from build123d import *

# Parameters (mm, degrees)
EXTRUDE_1_DEPTH     = 191
SKETCH_2_R          = 4.25
CUT_EXTRUDE_1_DEPTH = 21
SKETCH_3_R          = 2.25
CUT_EXTRUDE_2_DEPTH = 41


with BuildPart() as part:
    # Эскиз1 → Бобышка-Вытянуть1 (new body)
    with BuildSketch(Plane(origin=(0, 0, 0), x_dir=(1, 0, 0), z_dir=(0, 1, 0))):
        Polygon((0, 0), (0, 20), (2, 20), (2, 2), (40, 2), (40, 0), align=None)
    extrude(amount=EXTRUDE_1_DEPTH)

    # Эскиз2 → Вырез-Вытянуть1 (cut, through all)
    with BuildSketch(Plane.XY):
        with Locations((20, 165.5)):
            Circle(SKETCH_2_R)
        with Locations((20, 95.5)):
            Circle(SKETCH_2_R)
        with Locations((20, 25.5)):
            Circle(SKETCH_2_R)
    extrude(amount=-CUT_EXTRUDE_1_DEPTH, mode=Mode.SUBTRACT)

    # Эскиз3 → Вырез-Вытянуть2 (cut, through all)
    with BuildSketch(Plane.ZY):
        with Locations((-10, 12)):
            Circle(SKETCH_3_R)
        with Locations((-10, 179)):
            Circle(SKETCH_3_R)
    extrude(amount=-CUT_EXTRUDE_2_DEPTH, mode=Mode.SUBTRACT)


solid = part.part
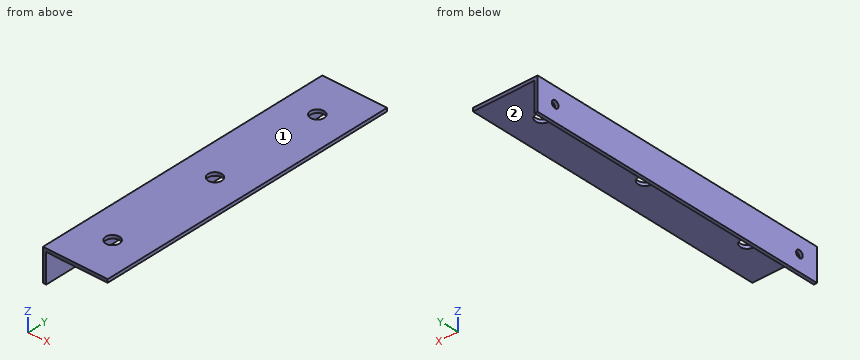
Geometry: final body of the model. Coordinates: model frame, mm. Face numbers are marked on the shaded views. A direction names the side the tool comes from. Coordinates: 2 decimals unless noted, no trailing zeros. Loops run counter-clockwise (first coordinate to the right, second up) from the corner with the lowest first, then second, coordinate; pieces in that order, holes last. Notation, with made-up numbers: M 2.25,-35.75 L 51.25,-35.75 A20 cw 51.25,-31.75 Z; hole C 60,0 d7. An arc over 180 degrees is marked long. One line per item, written item: value. Start each with the question number.
1) Pin query (flat end, axial travel): P1, Ø11, axis at x = 20, y = 25.5, coming from the -Z side; P2, Ø9, axis at y = 119.5, z = -12, coming from the +X side. Return the tip coordinate at first contact, or that it passes through.
2) Cut plane D-D (y = 88). Return loops of the section in (x, z), then the cut area to 3 significant figures.
3) Cut plane A-A (x = 20). Return loops of the section in (y, z).
4) Cut plane B-B (y = 179). Return loops of the section in (x, z), then the cut area to 3 significant figures.
5) Reachability of the marked faces 1 and 2 from +Z, -Z, +X, -X, +Y, -Y: full face, straight path, thin tool, end or side. Return the list, or none.
6) Material intervals for L1, parallel to Y at x = 1.35, z = -10; L2, parallel to Y at x = 20, z = -0.7; L3, parallel to X at y = 121, z = -17.25, sorted ascending. Write a range as from..to.
7) Cut plane C-C (z = -10). Return loops of the section in (x, y).
Evaluation:
1. P1: z = -2
1. P2: x = 2
2. outline: M 0,-20 L 2,-20 L 2,-2 L 40,-2 L 40,0 L 0,0 Z
2. area: 116 mm^2
3. outline: M 0,-2 L 21.25,-2 L 21.25,0 L 0,0 Z; M 29.75,-2 L 91.25,-2 L 91.25,0 L 29.75,0 Z; M 99.75,-2 L 161.25,-2 L 161.25,0 L 99.75,0 Z; M 169.75,-2 L 191,-2 L 191,0 L 169.75,0 Z
4. outline: M 0,-20 L 2,-20 L 2,-12.25 L 0,-12.25 Z; M 0,-7.75 L 2,-7.75 L 2,-2 L 40,-2 L 40,0 L 0,0 Z
4. area: 107 mm^2
5. face 1: +Z, +X, -X, +Y, -Y
5. face 2: -Z, +X, +Y, -Y
6. L1: 0..9.75, 14.25..176.75, 181.25..191
6. L2: 0..21.25, 29.75..91.25, 99.75..161.25, 169.75..191
6. L3: 0..2
7. outline: M 0,0 L 2,0 L 2,9.75 L 0,9.75 Z; M 0,14.25 L 2,14.25 L 2,176.75 L 0,176.75 Z; M 0,181.25 L 2,181.25 L 2,191 L 0,191 Z
